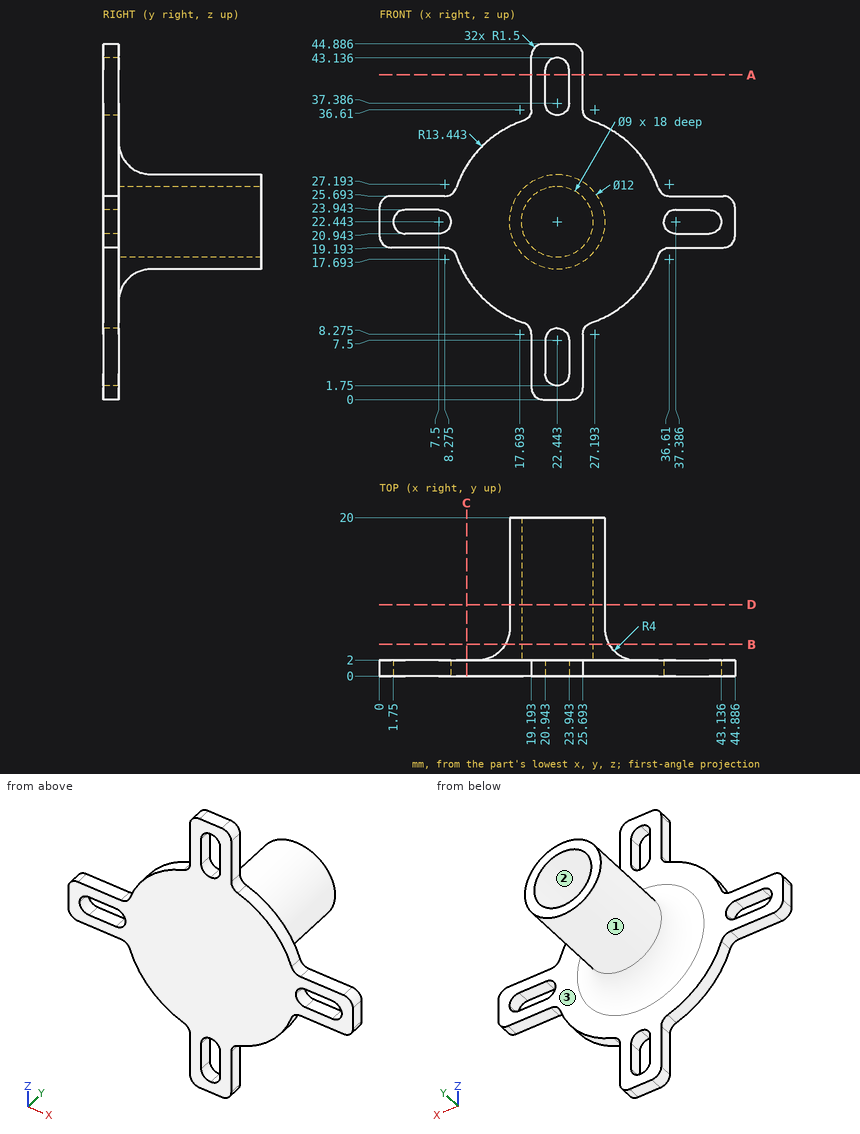
Check sheet for the drawn part. Datum: minimum x, y, z corner. Units: mm. Coordinates: 2 decimals unless noted, no trailing zeros. Order: outer loops, then holes, each group sorted by start corner. A loop starts at its lowest first (then second) coordinate and runs counter-clockwise, first axis right, second up. Notation, with made-up numbers: M -28.75,58 L 18.25,58 A20 ccw 18.25,81 Z; hole C 35,-8.75 d3. An arc over 180 degrees is marked long. One line per question, with ' | ' between items. Start each with the question number.
Item 1: Gauge pin test, flat ends, axial feed: P1, Ø12, axis at y = 10.5, z = 33.5, coming from the +X side; P2, Ø1.6, axis at y = 1, z = 4.5, coming from the -X side; P3, Ø0.6, axis at x = 6, y = 1.5, coming from the +Z side. Record the tip position at first contact, or that the pin passes through.
Item 2: Sectioned sample at B-B on y = 4. Record the cut outline in (x, z) (1 decimal).
Item 3: Sectioned sample at A-A on z = 41. Record the cut outline in (x, y).
Item 4: Sectioned sample at D-D on y = 9. Record the cut outline in (x, z).
Item 5: Sectioned sample at C-C on x = 11. Record the cut outline in (y, z).
Item 6: Material ranges on line 1 (Y direction, x = 43.5, z = 20); line 2 (Z direction, x = 22, y = 15.5) (1 decimal); line 3 (Z direction, x = 19.5, y = 4) (1 decimal), recorded low to high.
Item 7: Mould release check, pull along Z, two halves, no side actions. Record for the marked faces 1, 2 and 3: pulls with the +Z half, pulls with the -Z half, needs draft (parallel to the pull), parting line crosses it, or undercut.
Answer below:
1) P1: stops at x = 25.67 | P2: stops at x = 19.19 | P3: stops at z = 25.69
2) outline: C 22.4,22.4 d13.1; hole C 22.4,22.4 d9
3) outline: M 19.19,0 L 20.94,0 L 20.94,2 L 19.19,2 Z; M 23.94,0 L 25.69,0 L 25.69,2 L 23.94,2 Z
4) outline: C 22.44,22.44 d12; hole C 22.44,22.44 d9
5) outline: M 0,15.39 L 2,15.39 L 2,29.5 L 0,29.5 Z
6) line 1: y = 0 to 2 | line 2: z = 16.5 to 18, 26.9 to 28.4 | line 3: z = 16.6 to 19, 25.8 to 28.3
7) face 1: parting line crosses it | face 2: undercut | face 3: needs draft
